Could you check a few things on this drawing? It's one solid part, dimensions in mm from its lowest x, y, z. Coordinates: 2 decimals unless noted, no trailing zeros. Write each loop counter-clockwise with the first axis right and the second up, starting at its lowest first coordinate (ties: lowest second). Pieces come first, ordered by that corner, then holes. Notation, with made-up numbers: (-8.75, 7) - (11.25, 7) arc R21 ccw to (11.25, 31) - close; hole circle Ø9 at (12.25, 26.25). An arc over 180 degrees is marked (long way). Use one line per item in the form item = value. Start each with the question number.
(1) If we section it at C-C on x = 19: Please give me the cut outline in (y, z) (1 decimal).
(2) For pin 1 Ø1 at (x, y) = (49.5, 2.5) entering from +Z; pin 2 Ø8 at (x, z) = (31.5, 25.5) entering from -Y, each with a flat end and sliding along its axis, tell me the tip position at first contact or that it passes through.
(3) If we section it at A-A on z = 30.5: Please give me the cut outline in (x, y), then the cut area to 3 significant figures.
(4) If I drill on probe 1 along Z at (x, y) = (29, 3) (1 decimal); probe 2 along Z at (x, y) = (34.5, 5) (1 decimal); probe 3 along X at (y, z) = (2.7, 15) (1 decimal), over which ranges is the centre line in solid material (lowest first)? Write a range as from..to.
(5) If we section it at D-D on x = 30.5: Please give me the cut outline in (y, z) (1 decimal), then the cut area to 3 significant figures.
(6) If we section it at B-B on y = 0.8: Give the number of separate pieces and of enclosed holes in the cut face, then the cut area to 3 significant figures.
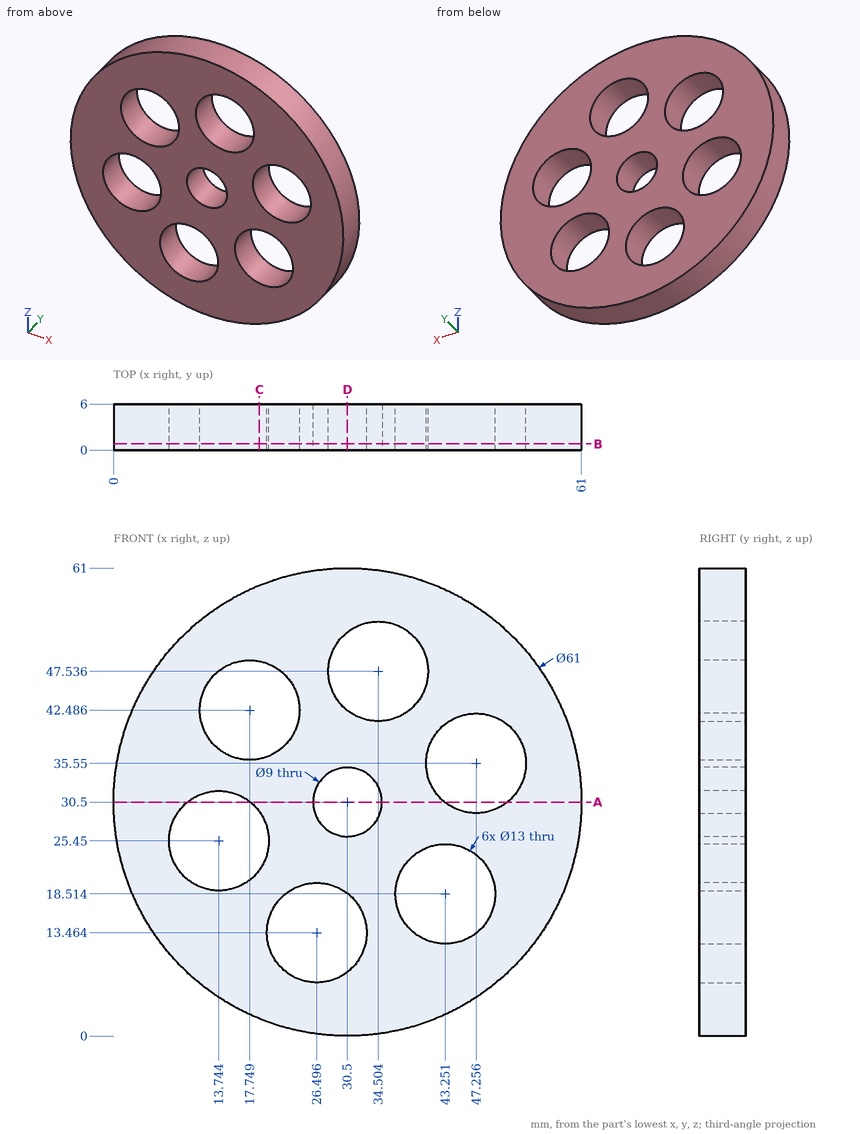
Reported:
q1.outline = (0, 2.3) - (6, 2.3) - (6, 21.6) - (0, 21.6) - close; (0, 29.3) - (6, 29.3) - (6, 36.1) - (0, 36.1) - close; (0, 48.9) - (6, 48.9) - (6, 58.7) - (0, 58.7) - close
q2.pin_1 = 54.75
q2.pin_2 = 0
q3.outline = (0, 0) - (9.65, 0) - (9.65, 6) - (0, 6) - close; (17.84, 0) - (26, 0) - (26, 6) - (17.84, 6) - close; (35, 0) - (43.16, 0) - (43.16, 6) - (35, 6) - close; (51.35, 0) - (61, 0) - (61, 6) - (51.35, 6) - close
q3.area = 214 mm2
q4.probe_1 = 0..7.5, 19.5..26.3, 34.7..44.1, 51..61
q4.probe_2 = 0.3..28.4, 32.6..41, 54..60.7
q4.probe_3 = 4.2..20.2, 32.8..37.8, 48.7..56.8
q5.outline = (0, 0) - (6, 0) - (6, 8.3) - (0, 8.3) - close; (0, 18.6) - (6, 18.6) - (6, 26) - (0, 26) - close; (0, 35) - (6, 35) - (6, 42.4) - (0, 42.4) - close; (0, 52.7) - (6, 52.7) - (6, 61) - (0, 61) - close
q5.area = 189 mm2
q6.separate_pieces = 1
q6.enclosed_holes = 7
q6.area = 2,060 mm2
